Read the model definition and answer for the solid it produces. Units are mm, in the model's axes. Face numbers are marked on the shaded views. A direction names the side the tool comes from. Round coordinates to 2 decimals unless told otherwise and drop trailing zeros. Order: outer loops, then holes, each group sorted by start corner. A loop starts at its lowest first (then second) coordinate and runs counter-clockwise, first axis right, second up. Notation, with made-up numbers: (40.5, 86.25) -> (66.5, 86.25) arc R9 ccw to (66.5, 96.25) -> close; hole circle Ø6 at (56.5, -5.5). An arc over 180 degrees is marked (long way). Use a Markdown table: item, result. Add a question column.
1. The mould has two halves that part along X. Classify the marked faces 1, 2, 3 and 4: +X half, -X half, draft (parallel to the pull), parting line (faces both ways), or undercut.
2. For the marked faces 5, 6 and 7, determine the directions among +Z, -Z, +X, -X, +Y, -Y from which every point of the face is accessible in a straight line to the end or side of a thin tool.
3. Section D-D, the plane x = 35.5 is taken. Give the vertices of the cut face in (y, z), then the cut area to 3 significant figures.
4. Given pin 1 (2.5 mm diameter, centred on x = -5, z = 5, fed in from +Y); pin 2 (8 mm diameter, centred on x = -12.5, y = 31, fed in from -Z); pin 3 (5 mm diameter, centred on x = 10, z = 95, fed in from +Y); pin 4 (4 mm diameter, centred on x = 13.31, y = 13.31, fed in from +Z), each flat-ended and moving along its own axis, determine where each tip first touches the part or whether it passes through.
5. Section B-B, the plane x = -5 is taken. Give the vertices of the cut face in (y, z), then the cut area to 3 significant figures.
6. Section C-C, the plane z = 41 is taken. Give the vertices of the cut face in (x, y).
7. Consider L1, parallel to X at y = 13, z = 64.5; L2, parallel to Y at x = -27.5, z = 87. Determine where each line is inside the solid, lowest interval first. Write a range as [from, to].
8. Section A-A, the plane y = 23 is taken. Give the vertices of the cut face in (x, z).
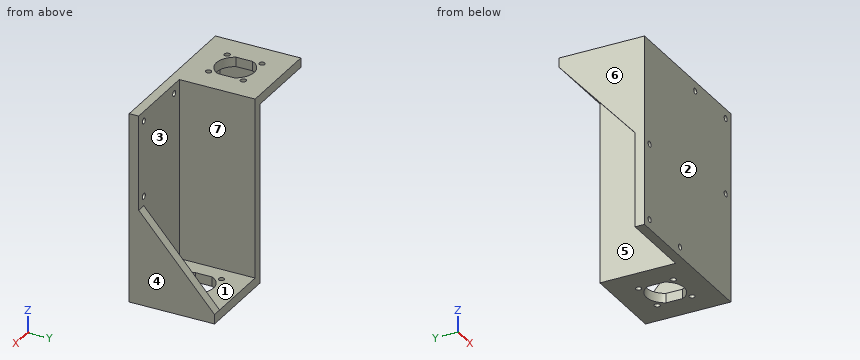
```python
from build123d import *

# Parameters (mm, degrees)
ESQUISSE1_W             = 45
ESQUISSE1_H             = 45
ESQUISSE1_R             = 1.5
EXTRUSION1_DEPTH        = 5
ESQUISSE2_W             = 45
ESQUISSE2_H             = 5
EXTRUSION2_DEPTH        = 95
EXTRUSION3_DEPTH        = 5
ESQUISSE4_W             = 95
ESQUISSE4_H             = 40
EXTRUSION4_DEPTH        = 5
ESQUISSE5_W             = 100
ESQUISSE5_H             = 5
EXTRUSION5_DEPTH        = 40
ESQUISSE6_W             = 40
ESQUISSE6_H             = 40
EXTRUSION6_DEPTH        = 5
EXTRUSION7_DEPTH        = 5
ENL_V_MAT_EXTRU_1_REACH = 102
ESQUISSE8_R             = 1.5
ENL_V_MAT_EXTRU_2_REACH = 7
ESQUISSE9_R             = 1.5


with BuildPart() as part:
    # Esquisse1 → Extrusion1 (new body)
    with BuildSketch(Plane.XY):
        with Locations((22.5, 22.5)):
            Rectangle(ESQUISSE1_W, ESQUISSE1_H)
        with Locations((31.692388155, 31.692388155)):
            Circle(ESQUISSE1_R, mode=Mode.SUBTRACT)
        with Locations((31.692388155, 13.307611845)):
            Circle(ESQUISSE1_R, mode=Mode.SUBTRACT)
        with Locations((13.307611845, 13.307611845)):
            Circle(ESQUISSE1_R, mode=Mode.SUBTRACT)
        with Locations((13.307611845, 31.692388155)):
            Circle(ESQUISSE1_R, mode=Mode.SUBTRACT)
        with BuildLine():
            Line((13.5, 26.858898944), (13.5, 18.141101056))
            ThreePointArc((13.5, 18.141101056), (22.5, 12.5), (31.5, 18.141101056))
            Line((31.5, 18.141101056), (31.5, 26.858898944))
            ThreePointArc((31.5, 26.858898944), (22.5, 32.5), (13.5, 26.858898944))
        make_face(mode=Mode.SUBTRACT)
    extrude(amount=EXTRUSION1_DEPTH)

    # Esquisse2 → Extrusion2 (add)
    with BuildSketch(Plane.XY.offset(5)):
        with Locations((22.5, 2.5)):
            Rectangle(ESQUISSE2_W, ESQUISSE2_H)
    extrude(amount=EXTRUSION2_DEPTH)

    # Esquisse3 → Extrusion3 (add)
    with BuildSketch(Plane(origin=(45, 0, 0), x_dir=(0, 0, -1), z_dir=(1, 0, 0))):
        Polygon((-5, 5), (-5, 45), (-50, 5), align=None)
    extrude(amount=-EXTRUSION3_DEPTH)

    # Esquisse4 → Extrusion4 (add)
    with BuildSketch(Plane.ZY):
        with Locations((52.5, 25)):
            Rectangle(ESQUISSE4_W, ESQUISSE4_H)
    extrude(amount=-EXTRUSION4_DEPTH)

    # Esquisse5 → Extrusion5 (add)
    with BuildSketch(Plane.ZY):
        with Locations((50, 2.5)):
            Rectangle(ESQUISSE5_W, ESQUISSE5_H)
    extrude(amount=EXTRUSION5_DEPTH)

    # Esquisse6 → Extrusion6 (add)
    with BuildSketch(Plane.XY.offset(100)):
        with Locations((-20, 25)):
            Rectangle(ESQUISSE6_W, ESQUISSE6_H)
    extrude(amount=-EXTRUSION6_DEPTH)

    # Esquisse7 → Extrusion7 (add)
    with BuildSketch(Plane.ZY.offset(40)):
        Polygon((95, 5), (95, 45), (50, 5), align=None)
    extrude(amount=-EXTRUSION7_DEPTH)

    # Esquisse8 → Enlèv. mat.-Extru.1 (cut, up to next)
    with BuildSketch(Plane.XY.offset(100), mode=Mode.PRIVATE) as enl_v_mat_extru_1_sk1:
        with Locations((-26.692388155, 31.692388155)):
            Circle(ESQUISSE8_R)
    enl_v_mat_extru_1_tool1 = extrude(enl_v_mat_extru_1_sk1.sketch, amount=-ENL_V_MAT_EXTRU_1_REACH, mode=Mode.PRIVATE) & part.part
    add(enl_v_mat_extru_1_tool1.solids().sort_by_distance((-26.692388, 31.692388, 100))[0], mode=Mode.SUBTRACT)
    # Esquisse8 → Enlèv. mat.-Extru.1 (cut, up to next)
    with BuildSketch(Plane.XY.offset(100), mode=Mode.PRIVATE) as enl_v_mat_extru_1_sk2:
        with Locations((-26.692388155, 13.307611845)):
            Circle(ESQUISSE8_R)
    enl_v_mat_extru_1_tool2 = extrude(enl_v_mat_extru_1_sk2.sketch, amount=-ENL_V_MAT_EXTRU_1_REACH, mode=Mode.PRIVATE) & part.part
    add(enl_v_mat_extru_1_tool2.solids().sort_by_distance((-26.692388, 13.307612, 100))[0], mode=Mode.SUBTRACT)
    # Esquisse8 → Enlèv. mat.-Extru.1 (cut, up to next)
    with BuildSketch(Plane.XY.offset(100), mode=Mode.PRIVATE) as enl_v_mat_extru_1_sk3:
        with Locations((-8.307611845, 13.307611845)):
            Circle(ESQUISSE8_R)
    enl_v_mat_extru_1_tool3 = extrude(enl_v_mat_extru_1_sk3.sketch, amount=-ENL_V_MAT_EXTRU_1_REACH, mode=Mode.PRIVATE) & part.part
    add(enl_v_mat_extru_1_tool3.solids().sort_by_distance((-8.307612, 13.307612, 100))[0], mode=Mode.SUBTRACT)
    # Esquisse8 → Enlèv. mat.-Extru.1 (cut, up to next)
    with BuildSketch(Plane.XY.offset(100), mode=Mode.PRIVATE) as enl_v_mat_extru_1_sk4:
        with Locations((-8.307611845, 31.692388155)):
            Circle(ESQUISSE8_R)
    enl_v_mat_extru_1_tool4 = extrude(enl_v_mat_extru_1_sk4.sketch, amount=-ENL_V_MAT_EXTRU_1_REACH, mode=Mode.PRIVATE) & part.part
    add(enl_v_mat_extru_1_tool4.solids().sort_by_distance((-8.307612, 31.692388, 100))[0], mode=Mode.SUBTRACT)
    # Esquisse8 → Enlèv. mat.-Extru.1 (cut, up to next)
    with BuildSketch(Plane.XY.offset(100), mode=Mode.PRIVATE) as enl_v_mat_extru_1_sk5:
        with BuildLine():
            Line((-26.5, 18.141101056), (-26.5, 26.858898944))
            ThreePointArc((-26.5, 26.858898944), (-17.5, 32.5), (-8.5, 26.858898944))
            Line((-8.5, 26.858898944), (-8.5, 18.141101056))
            ThreePointArc((-8.5, 18.141101056), (-17.5, 12.5), (-26.5, 18.141101056))
        make_face()
    enl_v_mat_extru_1_tool5 = extrude(enl_v_mat_extru_1_sk5.sketch, amount=-ENL_V_MAT_EXTRU_1_REACH, mode=Mode.PRIVATE) & part.part
    add(enl_v_mat_extru_1_tool5.solids().sort_by_distance((-17.5, 22.5, 100))[0], mode=Mode.SUBTRACT)

    # Esquisse9 → Enlèv. mat.-Extru.2 (cut, up to next)
    with BuildSketch(Plane(origin=(0, 5, 0), x_dir=(-1, 0, 0), z_dir=(0, 1, 0)), mode=Mode.PRIVATE) as enl_v_mat_extru_2_sk1:
        with Locations((-40, 95)):
            Circle(ESQUISSE9_R)
    enl_v_mat_extru_2_tool1 = extrude(enl_v_mat_extru_2_sk1.sketch, amount=-ENL_V_MAT_EXTRU_2_REACH, mode=Mode.PRIVATE) & part.part
    add(enl_v_mat_extru_2_tool1.solids().sort_by_distance((40, 5, 95))[0], mode=Mode.SUBTRACT)
    # Esquisse9 → Enlèv. mat.-Extru.2 (cut, up to next)
    with BuildSketch(Plane(origin=(0, 5, 0), x_dir=(-1, 0, 0), z_dir=(0, 1, 0)), mode=Mode.PRIVATE) as enl_v_mat_extru_2_sk2:
        with Locations((-10, 95)):
            Circle(ESQUISSE9_R)
    enl_v_mat_extru_2_tool2 = extrude(enl_v_mat_extru_2_sk2.sketch, amount=-ENL_V_MAT_EXTRU_2_REACH, mode=Mode.PRIVATE) & part.part
    add(enl_v_mat_extru_2_tool2.solids().sort_by_distance((10, 5, 95))[0], mode=Mode.SUBTRACT)
    # Esquisse9 → Enlèv. mat.-Extru.2 (cut, up to next)
    with BuildSketch(Plane(origin=(0, 5, 0), x_dir=(-1, 0, 0), z_dir=(0, 1, 0)), mode=Mode.PRIVATE) as enl_v_mat_extru_2_sk3:
        with Locations((35, 5)):
            Circle(ESQUISSE9_R)
    enl_v_mat_extru_2_tool3 = extrude(enl_v_mat_extru_2_sk3.sketch, amount=-ENL_V_MAT_EXTRU_2_REACH, mode=Mode.PRIVATE) & part.part
    add(enl_v_mat_extru_2_tool3.solids().sort_by_distance((-35, 5, 5))[0], mode=Mode.SUBTRACT)
    # Esquisse9 → Enlèv. mat.-Extru.2 (cut, up to next)
    with BuildSketch(Plane(origin=(0, 5, 0), x_dir=(-1, 0, 0), z_dir=(0, 1, 0)), mode=Mode.PRIVATE) as enl_v_mat_extru_2_sk4:
        with Locations((5, 5)):
            Circle(ESQUISSE9_R)
    enl_v_mat_extru_2_tool4 = extrude(enl_v_mat_extru_2_sk4.sketch, amount=-ENL_V_MAT_EXTRU_2_REACH, mode=Mode.PRIVATE) & part.part
    add(enl_v_mat_extru_2_tool4.solids().sort_by_distance((-5, 5, 5))[0], mode=Mode.SUBTRACT)
    # Esquisse9 → Enlèv. mat.-Extru.2 (cut, up to next)
    with BuildSketch(Plane(origin=(0, 5, 0), x_dir=(-1, 0, 0), z_dir=(0, 1, 0)), mode=Mode.PRIVATE) as enl_v_mat_extru_2_sk5:
        with Locations((-40, 55)):
            Circle(ESQUISSE9_R)
    enl_v_mat_extru_2_tool5 = extrude(enl_v_mat_extru_2_sk5.sketch, amount=-ENL_V_MAT_EXTRU_2_REACH, mode=Mode.PRIVATE) & part.part
    add(enl_v_mat_extru_2_tool5.solids().sort_by_distance((40, 5, 55))[0], mode=Mode.SUBTRACT)
    # Esquisse9 → Enlèv. mat.-Extru.2 (cut, up to next)
    with BuildSketch(Plane(origin=(0, 5, 0), x_dir=(-1, 0, 0), z_dir=(0, 1, 0)), mode=Mode.PRIVATE) as enl_v_mat_extru_2_sk6:
        with Locations((35, 45)):
            Circle(ESQUISSE9_R)
    enl_v_mat_extru_2_tool6 = extrude(enl_v_mat_extru_2_sk6.sketch, amount=-ENL_V_MAT_EXTRU_2_REACH, mode=Mode.PRIVATE) & part.part
    add(enl_v_mat_extru_2_tool6.solids().sort_by_distance((-35, 5, 45))[0], mode=Mode.SUBTRACT)


solid = part.part
```
Verdict:
| question | item | result |
|---|---|---|
| 1 | face 1 | undercut |
| 1 | face 2 | draft |
| 1 | face 3 | undercut |
| 1 | face 4 | +X half |
| 2 | face 5 | -Z, +Y |
| 2 | face 6 | +Z, -Z, -X, +Y, -Y |
| 2 | face 7 | +Z, +Y |
| 3 | outline | (0, 0) -> (45, 0) -> (45, 5) -> (5, 5) -> (5, 100) -> (0, 100) -> close |
| 3 | area | 700 mm2 |
| 4 | pin 1 | passes through |
| 4 | pin 2 | stops at z = 95 |
| 4 | pin 3 | stops at y = 5 |
| 4 | pin 4 | stops at z = 5 |
| 5 | outline | (0, 0) -> (5, 0) -> (5, 3.5) -> (0, 3.5) -> close; (0, 6.5) -> (5, 6.5) -> (5, 95) -> (45, 95) -> (45, 100) -> (0, 100) -> close |
| 5 | area | 685 mm2 |
| 6 | outline | (-40, 0) -> (45, 0) -> (45, 13) -> (40, 13) -> (40, 5) -> (5, 5) -> (5, 45) -> (0, 45) -> (0, 5) -> (-40, 5) -> close |
| 7 | L1 | x = [-40, -35], [0, 5] |
| 7 | L2 | y = [0, 5] |
| 8 | outline | (-40, 70.25) -> (-35, 70.25) -> (-35, 95) -> (-26.5, 95) -> (-26.5, 100) -> (-40, 100) -> close; (-8.5, 95) -> (0, 95) -> (0, 0) -> (13.5, 0) -> (13.5, 5) -> (5, 5) -> (5, 100) -> (-8.5, 100) -> close; (31.5, 0) -> (45, 0) -> (45, 29.75) -> (40, 29.75) -> (40, 5) -> (31.5, 5) -> close |
